Design review of the part built by this model. Coordinates are the model's own, in mm. A direction names the side the tool comes from. Give positions to 0.01 mm unless a question says otherwise; leave off trailing zeros. Write each loop counter-clockwise with the first axis right and the second up, starting at its lowest first coordinate (ties: lowest second). Pieces come first, ordered by that corner, then holes. Notation, with made-up numbers: M 25,77 L 74,77 A5 cw 74,84 Z; hole C 89,22.5 d7. An arc over 180 degrees is marked long. Answer in a Markdown table with one row per item.
```python
from build123d import *

# Parameters (mm, degrees)
F0_W     = 22
F0_H     = 1
F1_DEPTH = 1
F0_W_2   = 157
F2_DEPTH = 11
F3_R     = 0.5


with BuildPart() as f1:
    # F0 (on Top) → F1 (new body)
    with BuildSketch(Plane.XY):
        Polygon((95, -1), (-62, -1), (-62, -3), (6, -3), (28, -3), (95, -3), align=None)
        with Locations((17, -3.5)):
            Rectangle(F0_W, F0_H)
    extrude(amount=F1_DEPTH)

    # F0 (on Top) → F2 (join)
    with BuildSketch(Plane.XY):
        Polygon((6, -4), (5, -4), (5, -5), (29, -5), (29, -4), (28, -4), align=None)
        Polygon((6, -3), (-62, -3), (-62, -4), (5, -4), (6, -4), align=None)
        Polygon((95, -4), (95, -3), (28, -3), (28, -4), (29, -4), align=None)
        with Locations((16.5, -0.5)):
            Rectangle(F0_W_2, F0_H)
    extrude(amount=F2_DEPTH)

    # F3
    f3_edges = [f1.edges().sort_by_distance(p)[0] for p in [
        (17, -5, 0),
        (5, -4.5, 0),
        (-28.5, -4, 0),
        (62, -4, 0),
        (29, -4.5, 0),
        (16.5, 0, 0),
    ]]
    fillet(f3_edges, radius=F3_R)


solid = f1.part
```
1) To check wall thickness, follow probe 1 along Y at (x, z) = (-41, 2); probe 2 along Y at (x, z) = (11, 10.25); probe 3 along X at (y, z) = (-3.05, 1.5). State the ranges of each line that lie inside material, in increasing order. Write a range as [from, to].
Geometry says:
| item | result |
|---|---|
| probe 1 | [-4, -3], [-1, 0] |
| probe 2 | [-5, -4], [-1, 0] |
| probe 3 | [-62, 6], [28, 95] |
2) The part is to be moulded in two halves that separate along Y. For faces 5 (the face through (15, 0, 6)), 6 (the face through (62, -3, 6)), 7 (the face through (-28, -3, 6)), 8 (the face through (-29, -4, 6)), say which applies: released by +Y, released by -Y, zero draft, split by the parting line, or undercut.
Geometry says:
| item | result |
|---|---|
| face 5 | released by +Y |
| face 6 | undercut |
| face 7 | undercut |
| face 8 | released by -Y |
3) Add section B-B (x = 48). Write out the cut boundary in (y, z), and give its area (3 significant figures).
Geometry says:
| item | result |
|---|---|
| outline | M -4,0.5 A0.5 ccw -3.5,0 L -0.5,0 A0.5 ccw 0,0.5 L 0,11 L -1,11 L -1,1 L -3,1 L -3,11 L -4,11 Z |
| area | 23.9 mm^2 |
4) Insertion check: P1, Ø1, axis at x = -39.5, z = 6, coming from the -Y side; P2, Ø0.5, axis at y = -4.5, z = 4, coming from the +X side; P3, Ø0.5, axis at y = -4.5, z = 4, coming from the -X side. Each pin has a flat end and moves straight along its axis. Give the tip position at first contact, or say it passes through.
Geometry says:
| item | result |
|---|---|
| P1 | y = -4 |
| P2 | x = 29 |
| P3 | x = 5 |
5) For faces 1 (the face through (17, -4, 6)), 2 (the face through (15, -1, 6)), 3 (the face through (62, -4, 6)), 4 (the face through (-62, -3.3, 5.4)), list the 3-axis set-ups (+Z, -Z, +X, -X, +Y, -Y) from which the entire face can be reached by the end or side of a thin tool; tool diameter is ignored.
Geometry says:
| item | result |
|---|---|
| face 1 | +Z |
| face 2 | +Z, +X, -X |
| face 3 | +Z, -Z, +X, -Y |
| face 4 | +Z, -Z, -X, +Y, -Y |
6) Add section D-D (x = 16.5). Write out the cut boundary in (y, z).
Geometry says:
| item | result |
|---|---|
| outline | M -5,0.5 A0.5 ccw -4.5,0 L -0.5,0 A0.5 ccw 0,0.5 L 0,11 L -1,11 L -1,1 L -4,1 L -4,11 L -5,11 Z |
7) Add section A-A (z = 3). Write out the cut boundary in (x, y), and give its area (3 significant figures).
Geometry says:
| item | result |
|---|---|
| outline | M -62,-4 L 5,-4 L 5,-5 L 29,-5 L 29,-4 L 95,-4 L 95,-3 L 28,-3 L 28,-4 L 6,-4 L 6,-3 L -62,-3 Z; M -62,-1 L 95,-1 L 95,0 L -62,0 Z |
| area | 316 mm^2 |
8) Add section C-C (y = -2.2). Write out the cut boundary in (x, z), and give its area (3 significant figures).
Geometry says:
| item | result |
|---|---|
| outline | M -62,0 L 95,0 L 95,1 L -62,1 Z |
| area | 157 mm^2 |
